from build123d import *

# Parameters (mm, degrees)
BOSS_EXTRU_1_DEPTH        = 13
COQUE1_T                  = -5
COQUE1_THICKNESS_2_FACE_W = 90
COQUE1_THICKNESS_2_FACE_H = 65
COQUE1_THICKNESS_2_DEPTH  = 2
ENL_V_MAT_EXTRU_1_REACH   = 110.96
ESQUISSE2_R               = 2.5
ENL_V_MAT_EXTRU_2_REACH   = 95.396
ESQUISSE3_R               = 2.5
BOSS_EXTRU_2_DEPTH        = 10
ESQUISSE6_R               = 2.5
ESQUISSE6_R_2             = 5
ENL_V_MAT_EXTRU_3_DEPTH   = 3


with BuildPart() as part:
    # Esquisse1 → Boss.-Extru.1 (new body)
    with BuildSketch(Plane.XY):
        Polygon((44.118436308, 33.728448276), (54.118436308, 33.728448276), (54.118436308, 23.728448276), (54.118436308, -41.271551724), (-45.881563692, -41.271551724), (-45.881563692, 33.728448276), align=None)
    extrude(amount=BOSS_EXTRU_1_DEPTH)

    # Coque1
    coque1_openings = [part.faces().sort_by_distance(p)[0] for p in [
        (4.118436308, -3.771551724, 13),
    ]]
    offset(amount=COQUE1_T, openings=coque1_openings, kind=Kind.INTERSECTION)

    # Coque1 thickness 2 face (on inner face of the shell) → Coque1 thickness 2 (cut)
    with BuildSketch(Plane(origin=(4.118436308, -3.771551724, 5), x_dir=(-1, 0, 0), z_dir=(0, 0, -1))):
        Rectangle(COQUE1_THICKNESS_2_FACE_W, COQUE1_THICKNESS_2_FACE_H)
    extrude(amount=COQUE1_THICKNESS_2_DEPTH, mode=Mode.SUBTRACT)

    # Enlèv. mat.-Extru.1: up to this face of the body (flat: up to its plane)
    enl_v_mat_extru_1_end = Plane(part.part.faces().sort_by_distance((54.118436308, -3.771551724, 6.5))[0])
    # Esquisse2 → Enlèv. mat.-Extru.1 (cut, up to the picked face)
    with BuildSketch(Plane.ZY.offset(45.881563692), mode=Mode.PRIVATE) as enl_v_mat_extru_1_sk1:
        with Locations(Location((8, -16.271551724, 0), (0, 0, 270))):
            Circle(ESQUISSE2_R)
    enl_v_mat_extru_1_tool1 = split(extrude(enl_v_mat_extru_1_sk1.sketch, amount=-ENL_V_MAT_EXTRU_1_REACH, mode=Mode.PRIVATE), bisect_by=enl_v_mat_extru_1_end, keep=Keep.BOTH, mode=Mode.PRIVATE)
    # Esquisse2 → Enlèv. mat.-Extru.1 (cut, up to the picked face)
    with BuildSketch(Plane.ZY.offset(45.881563692), mode=Mode.PRIVATE) as enl_v_mat_extru_1_sk2:
        with Locations(Location((8, 8.728448276, 0), (0, 0, 270))):
            Circle(ESQUISSE2_R)
    enl_v_mat_extru_1_tool2 = split(extrude(enl_v_mat_extru_1_sk2.sketch, amount=-ENL_V_MAT_EXTRU_1_REACH, mode=Mode.PRIVATE), bisect_by=enl_v_mat_extru_1_end, keep=Keep.BOTH, mode=Mode.PRIVATE)
    add(enl_v_mat_extru_1_tool1.solids().sort_by(Axis((-45.881564, -16.271552, 8), (1, 0, 0)))[0], mode=Mode.SUBTRACT)
    add(enl_v_mat_extru_1_tool2.solids().sort_by(Axis((-45.881564, 8.728448, 8), (1, 0, 0)))[0], mode=Mode.SUBTRACT)

    # Enlèv. mat.-Extru.2: up to this face of the body (flat: up to its plane)
    enl_v_mat_extru_2_end = Plane(part.part.faces().sort_by_distance((4.118436308, 33.728448276, 6.5))[0])
    # Esquisse3 → Enlèv. mat.-Extru.2 (cut, up to the picked face)
    with BuildSketch(Plane.XZ.offset(41.271551724), mode=Mode.PRIVATE) as enl_v_mat_extru_2_sk1:
        with Locations(Location((-20.881563692, 8, 0), (0, 0, 270))):
            Circle(ESQUISSE3_R)
    enl_v_mat_extru_2_tool1 = split(extrude(enl_v_mat_extru_2_sk1.sketch, amount=-ENL_V_MAT_EXTRU_2_REACH, mode=Mode.PRIVATE), bisect_by=enl_v_mat_extru_2_end, keep=Keep.BOTH, mode=Mode.PRIVATE)
    # Esquisse3 → Enlèv. mat.-Extru.2 (cut, up to the picked face)
    with BuildSketch(Plane.XZ.offset(41.271551724), mode=Mode.PRIVATE) as enl_v_mat_extru_2_sk2:
        with Locations(Location((29.118436308, 8, 0), (0, 0, 270))):
            Circle(ESQUISSE3_R)
    enl_v_mat_extru_2_tool2 = split(extrude(enl_v_mat_extru_2_sk2.sketch, amount=-ENL_V_MAT_EXTRU_2_REACH, mode=Mode.PRIVATE), bisect_by=enl_v_mat_extru_2_end, keep=Keep.BOTH, mode=Mode.PRIVATE)
    add(enl_v_mat_extru_2_tool1.solids().sort_by(Axis((-20.881564, -41.271552, 8), (0, 1, 0)))[0], mode=Mode.SUBTRACT)
    add(enl_v_mat_extru_2_tool2.solids().sort_by(Axis((29.118436, -41.271552, 8), (0, 1, 0)))[0], mode=Mode.SUBTRACT)

    # Esquisse4 → Boss.-Extru.2 (add)
    with BuildSketch(Plane.XY.offset(3)):
        Polygon((-30.881563692, 28.728448276), (-40.881563692, 18.728448276), (-40.881563692, 28.728448276), align=None)
        Polygon((49.118436308, 28.728448276), (49.118436308, 18.728448276), (39.118436308, 28.728448276), align=None)
        Polygon((49.118436308, -36.271551724), (49.118436308, -26.271551724), (39.118436308, -36.271551724), align=None)
        Polygon((-30.881563692, -36.271551724), (-40.881563692, -26.271551724), (-40.881563692, -36.271551724), align=None)
    extrude(amount=BOSS_EXTRU_2_DEPTH)

    # Esquisse6 → Enlèv. mat.-Extru.3 (cut)
    with BuildSketch(Plane.XY.offset(3)):
        with Locations((-30.881563692, -21.271551724)):
            Circle(ESQUISSE6_R)
        with Locations((29.118436308, -21.271551724)):
            Circle(ESQUISSE6_R)
        with Locations((-30.881563692, 8.728448276)):
            Circle(ESQUISSE6_R)
        with Locations((29.118436308, 8.728448276)):
            Circle(ESQUISSE6_R)
        with Locations((39.118436308, 19.605642263)):
            Circle(ESQUISSE6_R_2)
    extrude(amount=-ENL_V_MAT_EXTRU_3_DEPTH, mode=Mode.SUBTRACT)


solid = part.part
Model file for the job. Use its own axes, mm. A direction names the side the tool comes from. Coordinates: 2 decimals unless noted, no trailing zeros. Write each loop counter-clockwise with the first axis right and the second up, starting at its lowest first coordinate (ties: lowest second). Pieces come first, ordered by that corner, then holes. Notation, with made-up numbers: (73.25, -27.5) - (80.25, -27.5) arc R27 cw to (80.25, 4.5) - close; hole circle Ø2 at (87, -10.75). An arc over 180 degrees is marked (long way). Write each question's results on one line, items separated by ' | '. Start each with the question number.
1) Cut at C-C (y = -32). Write the cut outline in (x, z).
2) Cut at D-D (z = 1.5). Write the cut outline in (x, y).
3) 3-axis set-ups, long thin cutter, end or side, ignore diameter. For faces 1 (the face through (31.6, 31.2, 8.3)), 2 (the face through (-40.882, -4, 8)): which of +Z, -Z, +X, -X, +Y, -Y reach the whole face in a straight line?
4) Cut at A-A (z = 8). Count the separate pieces of the cut face and the enclosed holes in it, then the cut area to 3 significant figures.
5) Probe line 1 along X through (y, z) = (-37.4, 8); line 2 along Y through (x, z) = (1, 10.75); line 3 along X through (y, z) = (2.5, 6.5). List the from-to ranges inside material, lowest first. Write a range as from..to.
6) Cut at B-B (x = -10). Write the cut outline in (y, z), then the cut area to 3 significant figures.
7) Flat gauge pin, fed straight in: P1, Ø8, axis at x = 29.12, y = 8.73, coming from the +Z side. Where does the tip first touch, or does it go through?
8) Mould opens along Y. For faces 3 (the face through (5, 33.728, 6)), 4 (the face through (-43.417, 7.575, 5.782)), 5 (the face through (54.118, -4, 6)) say: pulls with the +Y half, pulls with the -Y half, needs draft (parallel to the pull), parting line crosses it, or undercut.
Returned:
1) outline: (-45.88, 0) - (54.12, 0) - (54.12, 13) - (43.39, 13) - (43.39, 3) - (-35.15, 3) - (-35.15, 13) - (-45.88, 13) - close
2) outline: (-45.88, -41.27) - (54.12, -41.27) - (54.12, 33.73) - (-45.88, 33.73) - close; hole circle Ø5 at (-30.88, -21.27); hole circle Ø5 at (-30.88, 8.73); hole circle Ø5 at (29.12, -21.27); hole circle Ø5 at (29.12, 8.73); hole circle Ø10 at (39.12, 19.61)
3) face 1: +Y, -Y | face 2: +Z
4) separate pieces: 8 | enclosed holes: 0 | area: 1,650 mm^2
5) line 1: -45.88..-23.38, -18.38..26.62, 31.62..54.12 | line 2: -41.27..-36.27, 28.73..33.73 | line 3: -45.88..-40.88, 49.12..54.12
6) outline: (-41.27, 0) - (33.73, 0) - (33.73, 13) - (28.73, 13) - (28.73, 3) - (-36.27, 3) - (-36.27, 13) - (-41.27, 13) - close | area: 325 mm^2
7) P1: z = 3
8) face 3: pulls with the +Y half | face 4: undercut | face 5: needs draft
